Check sheet for the modelled part. Datum: model origin and axes. Units: mm. Face numbers are marked on the shaded views. Coordinates: 2 decimals unless noted, no trailing zeros. Order: outer loops, then holes, each group sorted by start corner. A loop starts at its lowest first (then second) coordinate and runs counter-clockwise, first axis right, second up.
1. Cross-section at B-B (x = -2). Enter the section's corners in (y, z).
2. Draft check along Z on the marked faces 1 and 2. Enter one of: released by +Z, released by -Z, zero draft, split by the parting line, or undercut.
3. Cross-section at A-A (y = -5.25). Enter the section's corners in (x, z), then the cut area to 3 significant figures.
4. Gauge pin test, flat ends, axial feed: pin 1 Ø4 at (x, z) = (-2, -41) entering from -Y; pin 2 Ø0.6 at (y, z) = (-4.5, -16.5) entering from -X; pin 3 Ø5 at (x, z) = (-12, -22) entering from +Y. Record the tip position at first contact, or that the pin passes through.
5. Cross-section at D-D (z = -4.5). Enter the section's corners in (x, y), then the cut area to 3 significant figures.
6. Thickness scan on line 1 (Z direction, x = -70, y = 0.2); line 2 (X direction, y = 0.5, z = -2); line 3 (Z direction, x = -69, y = -1). Record the ranges inside material, lowest first.
7. Cross-section at C-C (y = 2). Enter the section's corners in (x, z).
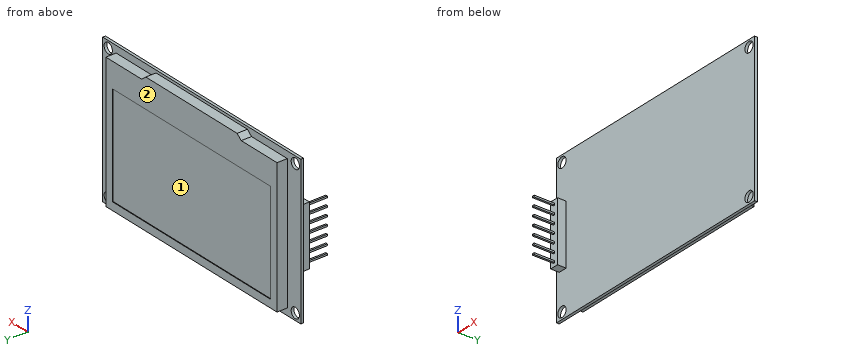
```python
from build123d import *

# Parameters (mm, degrees)
SKETCH1_W           = 72
SKETCH1_H           = 43
SKETCH1_R           = 1.5
BOSS_EXTRUDE1_DEPTH = 0.8
SKETCH2_W           = 62.2
SKETCH2_H           = 39
SKETCH2_W_2         = 33.2
SKETCH2_H_2         = 1.237316914
BOSS_EXTRUDE2_DEPTH = 3
SKETCH3_W           = 57.5
SKETCH3_H           = 29.5
CUT_EXTRUDE1_DEPTH  = 0.2
SKETCH4_W           = 2.5
SKETCH4_H           = 17.5
BOSS_EXTRUDE3_DEPTH = 2.5
SKETCH5_W           = 0.5
SKETCH5_H           = 0.5
BOSS_EXTRUDE4_DEPTH = 6
LPATTERN1_COUNT     = 7
LPATTERN1_PITCH     = 2.5


with BuildPart() as part:
    # Sketch1 → Boss-Extrude1 (new body)
    with BuildSketch(Plane(origin=(0, 0, 0), x_dir=(1, 0, 0), z_dir=(0, 1, 0))):
        with Locations((-36, 21.5)):
            Rectangle(SKETCH1_W, SKETCH1_H)
        with Locations(Location((-70, 41, 0), (0, 0, 270))):
            Circle(SKETCH1_R, mode=Mode.SUBTRACT)
        with Locations(Location((-2, 41, 0), (0, 0, 270))):
            Circle(SKETCH1_R, mode=Mode.SUBTRACT)
        with Locations(Location((-2, 2, 0), (0, 0, 270))):
            Circle(SKETCH1_R, mode=Mode.SUBTRACT)
        with Locations(Location((-70, 2, 0), (0, 0, 270))):
            Circle(SKETCH1_R, mode=Mode.SUBTRACT)
    extrude(amount=BOSS_EXTRUDE1_DEPTH)

    # Sketch2 → Boss-Extrude2 (add)
    with BuildSketch(Plane(origin=(0, 0.8, 0), x_dir=(1, 0, 0), z_dir=(0, 1, 0))):
        with Locations((-36, 21.5)):
            Rectangle(SKETCH2_W, SKETCH2_H)
        with Locations((-36, 1.381341543)):
            Rectangle(SKETCH2_W_2, SKETCH2_H_2)
        Polygon((-19.4, 0.762683086), (-17.9, 2), (-19.4, 2), align=None)
        Polygon((-52.6, 2), (-54.1, 2), (-52.6, 0.762683086), align=None)
    extrude(amount=BOSS_EXTRUDE2_DEPTH)

    # Sketch3 → Cut-Extrude1 (cut)
    with BuildSketch(Plane(origin=(0, 3.8, 0), x_dir=(1, 0, 0), z_dir=(0, 1, 0))):
        with Locations((-36, 23.95)):
            Rectangle(SKETCH3_W, SKETCH3_H)
    extrude(amount=-CUT_EXTRUDE1_DEPTH, mode=Mode.SUBTRACT)

    # Sketch4 → Boss-Extrude3 (add)
    with BuildSketch(Plane.XZ):
        with Locations((-69.75, -21.5)):
            Rectangle(SKETCH4_W, SKETCH4_H)
    extrude(amount=BOSS_EXTRUDE3_DEPTH)

    # Sketch5 → Boss-Extrude4 (add)
    with BuildSketch(Plane.XZ.offset(2.5)):
        with Locations((-69.75, -14)):
            Rectangle(SKETCH5_W, SKETCH5_H)
    boss_extrude4 = extrude(amount=BOSS_EXTRUDE4_DEPTH)

    # LPattern1: Boss-Extrude4 ×7
    with Locations(*[(0, 0, -i * LPATTERN1_PITCH) for i in range(1, LPATTERN1_COUNT)]):
        add(boss_extrude4)


solid = part.part
```
Data:
1. outline: (0, -43) - (0.8, -43) - (0.8, -42.5) - (0, -42.5) - close; (0, -39.5) - (0.8, -39.5) - (0.8, -3.5) - (0, -3.5) - close; (0, -0.5) - (0.8, -0.5) - (0.8, 0) - (0, 0) - close
2. face 1: undercut
2. face 2: zero draft
3. outline: (-70, -29.25) - (-69.5, -29.25) - (-69.5, -28.75) - (-70, -28.75) - close; (-70, -26.75) - (-69.5, -26.75) - (-69.5, -26.25) - (-70, -26.25) - close; (-70, -24.25) - (-69.5, -24.25) - (-69.5, -23.75) - (-70, -23.75) - close; (-70, -21.75) - (-69.5, -21.75) - (-69.5, -21.25) - (-70, -21.25) - close; (-70, -19.25) - (-69.5, -19.25) - (-69.5, -18.75) - (-70, -18.75) - close; (-70, -16.75) - (-69.5, -16.75) - (-69.5, -16.25) - (-70, -16.25) - close; (-70, -14.25) - (-69.5, -14.25) - (-69.5, -13.75) - (-70, -13.75) - close
3. area: 1.75 mm2
4. pin 1: stops at y = 0
4. pin 2: stops at x = -70
4. pin 3: stops at y = 3.6
5. outline: (-72, 0) - (0, 0) - (0, 0.8) - (-4.9, 0.8) - (-4.9, 3.8) - (-67.1, 3.8) - (-67.1, 0.8) - (-72, 0.8) - close
5. area: 244 mm2
6. line 1: z = -43 to -42.5, -39.5 to -3.5, -0.5 to 0
6. line 2: x = -72 to -71.5, -68.5 to -3.5, -0.5 to 0
6. line 3: z = -30.25 to -12.75
7. outline: (-67.1, -41) - (-4.9, -41) - (-4.9, -2) - (-17.9, -2) - (-19.4, -0.76) - (-52.6, -0.76) - (-54.1, -2) - (-67.1, -2) - close
